from build123d import *

# Parameters (mm, degrees)
SKETCH1_R           = 1.5
BOSS_EXTRUDE1_DEPTH = 25
SKETCH2_R           = 2.6
BOSS_EXTRUDE2_DEPTH = 1.7
BOSS_EXTRUDE2_TAPER = 32
SKETCH3_W           = 0.5
SKETCH3_H           = 1.758378485
SKETCH3_H_2         = 1.741621515
SKETCH3_W_2         = 1.734727157
SKETCH3_H_3         = 0.5
SKETCH3_W_3         = 1.765272843
CUT_EXTRUDE1_DEPTH  = 0.3


with BuildPart() as part:
    # Sketch1 → Boss-Extrude1 (new body)
    with BuildSketch(Plane(origin=(0, 0, 0), x_dir=(1, 0, 0), z_dir=(0, 1, 0))):
        Circle(SKETCH1_R)
    extrude(amount=BOSS_EXTRUDE1_DEPTH)

    # Sketch2 → Boss-Extrude2 (add)
    with BuildSketch(Plane(origin=(0, 25, 0), x_dir=(1, 0, 0), z_dir=(0, 1, 0))):
        Circle(SKETCH2_R)
    extrude(amount=-BOSS_EXTRUDE2_DEPTH, taper=BOSS_EXTRUDE2_TAPER)

    # Sketch3 → Cut-Extrude1 (cut)
    with BuildSketch(Plane(origin=(0, 25, 0), x_dir=(1, 0, 0), z_dir=(0, 1, 0))):
        with Locations((-0.015272843, 1.120810757)):
            Rectangle(SKETCH3_W, SKETCH3_H)
        with Locations((-0.015272843, -1.129189243)):
            Rectangle(SKETCH3_W, SKETCH3_H_2)
        with Locations((-1.132636421, -0.008378485)):
            Rectangle(SKETCH3_W_2, SKETCH3_H_3)
        with Locations((1.117363579, -0.008378485)):
            Rectangle(SKETCH3_W_3, SKETCH3_H_3)
        with Locations((-0.015272843, -0.008378485)):
            Rectangle(SKETCH3_W, SKETCH3_H_3)
    extrude(amount=-CUT_EXTRUDE1_DEPTH, mode=Mode.SUBTRACT)


solid = part.part
Model file for the job. Use its own axes, mm. A direction names the side the tool comes from. Give positions to 0.01 mm unless a question says otherwise; leave off trailing zeros. Order: outer loops, then holes, each group sorted by start corner. A loop starts at its lowest first (then second) coordinate and runs counter-clockwise, first axis right, second up. Notation, with made-up numbers: (11, 86) - (56, 86) arc R34 ccw to (56, 124) - close; hole circle Ø9 at (68, 4). An arc over 180 degrees is marked (long way). Return JSON: item names as keys, results as strings.
1) Flat gauge pins, fed straight in: P1, Ø3, axis at y = 11.5, z = -1.5, coming from the -X side; P2, Ø1, axis at x = -0.5, y = 9.5, coming from the +Z side; P3, Ø3, axis at x = 0, z = 0, coming from the +Y side. Where does each tip first touch, or does it go through?
Geometry says:
{"P1": "x = -1.5", "P2": "z = 1.5", "P3": "y = 25"}
2) 3-axis set-ups, long thin cutter, end or side, ignore diameter. For faces 1 (the cylindrical face through (-1.5, 11.49, -0.07)), 2 (the flat face through (0, 0, 0)): which of +Z, -Z, +X, -X, +Y, -Y reach the whole face in a straight line?
Geometry says:
{"face 1": "-Y", "face 2": "+Z, -Z, +X, -X, -Y"}
3) Cut at B-B, the plane y = 21.5. Give the cut face in (x, z).
Geometry says:
{"outline": "circle Ø3 at (0, 0)"}
4) Probe line 1 (Y direction, x = -0.2, z = 1.3); line 2 (Y direction, x = -0.2, z = 2.4); line 3 (Z direction, x = -0.1, y = 22.5). List the from-to ranges inside material, lowest first. Write a range as from..to.
Geometry says:
{"line 1": "0..24.7", "line 2": "24.69..25", "line 3": "-1.5..1.5"}
